The figure shows three views and two pictorial views of one solid part (mm, origin at its lowest corner). Answer the questions. Coordinates: 2 decimals unless noted, no trailing zeros. Order: outer loops, then holes, each group sorted by start corner. A loop starts at its lowest first (then second) coordinate and runs counter-clockwise, first axis right, second up.
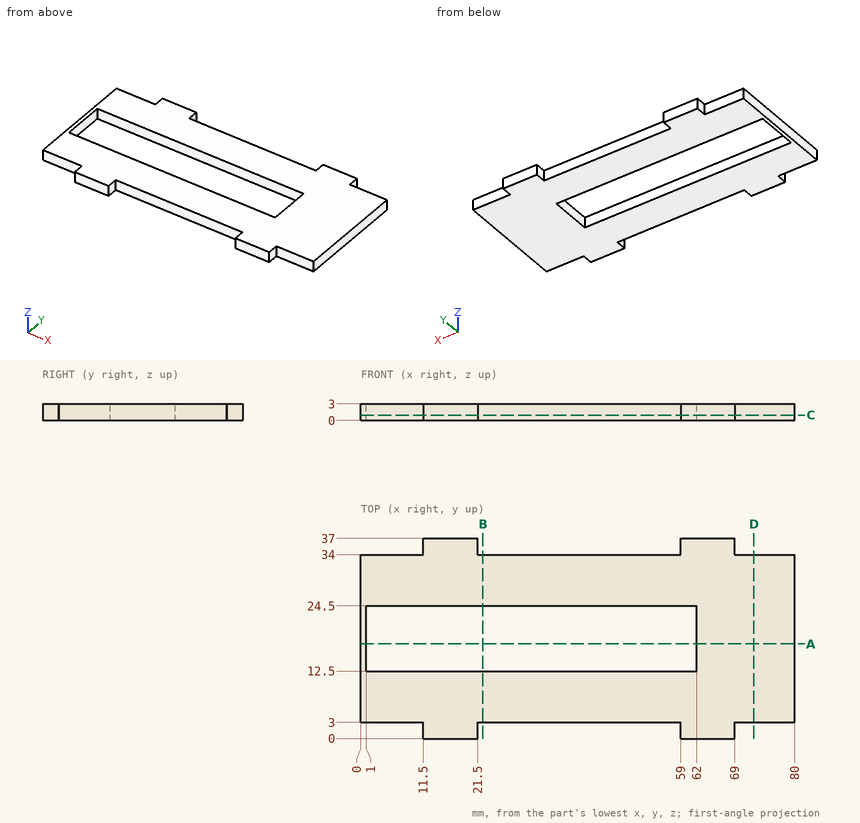
1) A cutting plane is placed at B-B, the plane x = 22.5. Write down the section's boundary in (y, z), plus the area to 3 significant figures.
2) Each of these flat-tipped pins is pushed along its axis until it touches: P1, Ø2, axis at x = 11.5, y = 6.5, coming from the -Z side; P2, Ø1.5, axis at y = 35, z = 2, coming from the -X side; P3, Ø0.9, axis at x = 31, z = 1.5, coming from the -Y side; P4, Ø1.5, axis at x = 3.5, z = 2, coming from the +Y side. Where does it stop, or does it pass through?
3) A cutting plane is placed at C-C, the plane z = 0.95. Write down the section's boundary in (x, y), plus the area to 3 significant figures.
4) A cutting plane is placed at A-A, the plane y = 17.5. Write down the section's boundary in (x, z), plus the area to 3 significant figures.
5) A cutting plane is placed at D-D, the plane x = 72.5. Write down the section's boundary in (y, z).
6) Straight lines are drawn through the part: probe 1 along X at (y, z) = (22.5, 0.3); probe 2 along Y at (x, z) = (10, 2.85); probe 3 along Y at (x, z) = (74, 0.3). For each, find the intervals that lie inside material, in ascending order.
Working result:
1. outline: (3, 0) - (12.5, 0) - (12.5, 3) - (3, 3) - close; (24.5, 0) - (34, 0) - (34, 3) - (24.5, 3) - close
1. area: 57.0 mm2
2. P1: stops at z = 0
2. P2: stops at x = 11.5
2. P3: stops at y = 3
2. P4: stops at y = 34
3. outline: (0, 3) - (11.5, 3) - (11.5, 0) - (21.5, 0) - (21.5, 3) - (59, 3) - (59, 0) - (69, 0) - (69, 3) - (80, 3) - (80, 34) - (69, 34) - (69, 37) - (59, 37) - (59, 34) - (21.5, 34) - (21.5, 37) - (11.5, 37) - (11.5, 34) - (0, 34) - close; hole (1, 12.5) - (62, 12.5) - (62, 24.5) - (1, 24.5) - close
3. area: 1,870 mm2
4. outline: (0, 0) - (1, 0) - (1, 3) - (0, 3) - close; (62, 0) - (80, 0) - (80, 3) - (62, 3) - close
4. area: 57.0 mm2
5. outline: (3, 0) - (34, 0) - (34, 3) - (3, 3) - close
6. probe 1: x = 0 to 1, 62 to 80
6. probe 2: y = 3 to 12.5, 24.5 to 34
6. probe 3: y = 3 to 34
